Could you check a few things on this drawing? It's one solid part, dimensions in mm from its lowest x, y, z. Coordinates: 2 decimals unless noted, no trailing zeros. Loops run counter-clockwise (first coordinate to the right, second up) from the corner with the lowest first, then second, coordinate; pieces in that order, holes last. Notation, with made-up numbers: M 8,72.25 L 35,72.25 A19 cw 35,81.25 Z; hole C -35,-3 d11. An arc over 180 degrees is marked long. Answer as a JSON object with one key per item and string values. Group by question number.
Item 1: We'd pull the mould along Y, two halves only. Please class the marked faces 1, 2, 3 and 4: +Y half, -Y half, draft (parallel to the pull), parting line (faces both ways), or undercut.
Item 2: Suppose I cut it at C-C (z = 8.75). Write out the boundary of the cut face in (x, y).
Item 3: Suppose I cut it at B-B (y = 25.4). Write out the boundary of the cut face in (x, z).
Item 4: Suppose I cut it at A-A (x = 38.1). Write out the boundary of the cut face in (y, z), then the cut area to 3 significant figures.
Item 5: If I drill on line 1 (X direction, y = 25.4, z = 3); line 2 (Y direction, x = 38.1, z = 8.25); line 3 (X direction, y = 21, z = 1), over which ranges is the centre line in solid material (lowest first)?
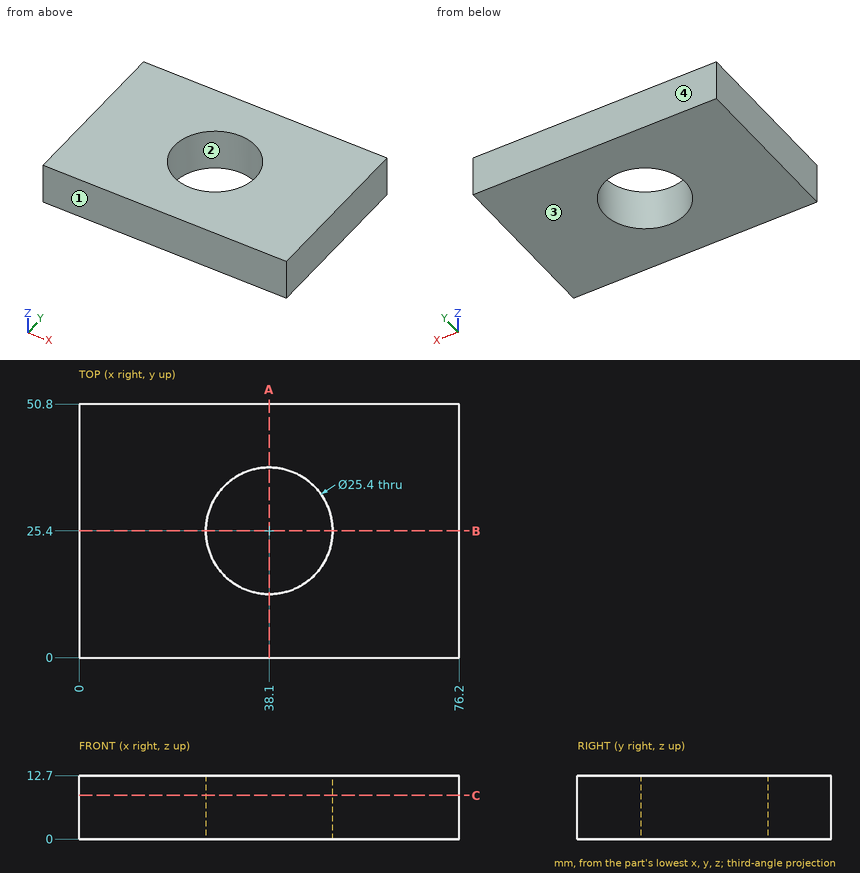
From the geometry:
{
 "1": {"face 1": "-Y half", "face 2": "undercut", "face 3": "draft", "face 4": "+Y half"},
 "2": {"outline": "M 0,0 L 76.2,0 L 76.2,50.8 L 0,50.8 Z; hole C 38.1,25.4 d25.4"},
 "3": {"outline": "M 0,0 L 25.4,0 L 25.4,12.7 L 0,12.7 Z; M 50.8,0 L 76.2,0 L 76.2,12.7 L 50.8,12.7 Z"},
 "4": {"outline": "M 0,0 L 12.7,0 L 12.7,12.7 L 0,12.7 Z; M 38.1,0 L 50.8,0 L 50.8,12.7 L 38.1,12.7 Z", "area": "323 mm2"},
 "5": {"line 1": "0 to 25.4, 50.8 to 76.2", "line 2": "0 to 12.7, 38.1 to 50.8", "line 3": "0 to 26.19, 50.01 to 76.2"}
}
